Geometry check sheet. Reference: the model listing, model coordinates, mm. A direction names the side the tool comes from. Round coordinates to 2 decimals unless told otherwise and drop trailing zeros. Write each loop counter-clockwise with the first axis right and the second up, starting at its lowest first coordinate (ties: lowest second). Pieces come first, ordered by that corner, then holes. Notation, with made-up numbers: (67, 82) -> (102, 82) arc R6 ccw to (102, 88) -> close; hole circle Ø4 at (-32, 12). An arc over 180 degrees is marked (long way). Use a Markdown table: item, result.
```python
from build123d import *

# Parameters (mm, degrees)
F1_W     = 163
F1_H     = 95.5
F2_DEPTH = 12.5


with BuildPart() as f2:
    # F1 (on Top) → F2 (new body)
    with BuildSketch(Plane.XY):
        Rectangle(F1_W, F1_H)
        with BuildLine():
            ThreePointArc((-56.5, 19.75), (-54.1568542495, 25.4068542495), (-48.5, 27.75))
            Line((-48.5, 27.75), (48.5, 27.75))
            ThreePointArc((48.5, 27.75), (54.1568542495, 25.4068542495), (56.5, 19.75))
            Line((56.5, 19.75), (56.5, -19.75))
            ThreePointArc((56.5, -19.75), (54.1568542495, -25.4068542495), (48.5, -27.75))
            Line((48.5, -27.75), (-48.5, -27.75))
            ThreePointArc((-48.5, -27.75), (-54.1568542495, -25.4068542495), (-56.5, -19.75))
            Line((-56.5, -19.75), (-56.5, 19.75))
        make_face(mode=Mode.SUBTRACT)
    extrude(amount=-F2_DEPTH)


solid = f2.part
```
(1) Access from +Z, -Z, +X, -X, +Y, -Y to the whole of each face (thin tool, end or side, straight path). Record for faces 4 (the face through (-1, 33, -12.5)), 5 (the face through (-54.094, -25.469, -6.162)).
A:
| item | result |
|---|---|
| face 4 | -Z, +X, -X, +Y, -Y |
| face 5 | +Z, -Z |
(2) Release check for a two-part mould opening along X. For faces 1 (the face through (-56.5, 0, -6)), 2 (the face through (-81.5, -1, -6)), 3 (the face through (-1, 33, 0)) record: +X half, -X half, draft (parallel to the pull), parting line (faces both ways), or undercut.
A:
| item | result |
|---|---|
| face 1 | undercut |
| face 2 | -X half |
| face 3 | draft |
(3) Section check A-A on x = -17. Record the cut outline in (y, z), plus the area to 3 significant figures.
A:
| item | result |
|---|---|
| outline | (-47.75, -12.5) -> (-27.75, -12.5) -> (-27.75, 0) -> (-47.75, 0) -> close; (27.75, -12.5) -> (47.75, -12.5) -> (47.75, 0) -> (27.75, 0) -> close |
| area | 500 mm2 |
(4) Thickness scan on line 1 (X direction, y = -1, z = -11); line 2 (Y direction, x = -21, z = -1); line 3 (Y direction, x = 52.5, z = -10.25). Record the ranges inside material, lowest first.
A:
| item | result |
|---|---|
| line 1 | x = -81.5 to -56.5, 56.5 to 81.5 |
| line 2 | y = -47.75 to -27.75, 27.75 to 47.75 |
| line 3 | y = -47.75 to -26.68, 26.68 to 47.75 |
(5) Section check B-B on y = 11. Record the cut outline in (x, z), plus the area to 3 significant figures.
A:
| item | result |
|---|---|
| outline | (-81.5, -12.5) -> (-56.5, -12.5) -> (-56.5, 0) -> (-81.5, 0) -> close; (56.5, -12.5) -> (81.5, -12.5) -> (81.5, 0) -> (56.5, 0) -> close |
| area | 625 mm2 |
(6) Section check C-C on z = -2. Record the cut outline in (x, y), plus the area to 3 significant figures.
A:
| item | result |
|---|---|
| outline | (-81.5, -47.75) -> (81.5, -47.75) -> (81.5, 47.75) -> (-81.5, 47.75) -> close; hole (-56.5, -19.75) arc R8 ccw to (-48.5, -27.75) -> (48.5, -27.75) arc R8 ccw to (56.5, -19.75) -> (56.5, 19.75) arc R8 ccw to (48.5, 27.75) -> (-48.5, 27.75) arc R8 ccw to (-56.5, 19.75) -> close |
| area | 9,350 mm2 |
